Input: part model. Units: mm. Frame: model coordinates. Face numbers are marked on the shaded views. A direction names the side the tool comes from. Coordinates: 2 decimals unless noted, no trailing zeros. Loops run counter-clockwise (first coordinate to the right, second up) from the corner with the lowest first, then second, coordinate; pieces in that order, holes last. Notation, with made-up numbers: (14.25, 26) -> (42.25, 26) arc R30 cw to (42.25, 56) -> close; hole circle Ø1 at (-17, -35). An arc over 180 degrees is marked (long way). Put each result on its own line as item: value. Start each with the question number.
1) Cut plane A-A (x = -4.5). Return the cut outline in (y, z).
2) Set-up query: the marked faces 1, 2 and 3. Return all of +Z, -Z, +X, -X, +Y, -Y with unobstructed straight access to the full face (end or side cutting, diameter ignored); none if empty.
3) Material intervals for L1, parallel to Z at x = -5.5, y = 10.5; L2, parallel to Y at x = 13, z = 2; L3, parallel to Z at x = 7, y = 4, sorted ascending.
4) Cut plane C-C (z = 44). Return the cut outline in (x, y).
5) Cut plane D-D (z = 76). Return the cut outline in (x, y).
6) Contact query for flat-ended pins moving along their axis: P1, Ø12, axis at x = 10, z = 90.5, coming from the +Y side; P2, Ø6, axis at x = 5, y = -4, coming from the -Z side; P3, Ø16, axis at x = -4.5, y = 2, coming from the -Z side; P4, Ø2, axis at y = -3, z = 20.5, coming from the -X side. Output: stop coordinate, or through.
7) Cut plane B-B (y = -5). Return the cut outline in (x, z), plus the area to 3 significant figures.
from build123d import *

# Parameters (mm, degrees)
SKETCH1_R           = 16
BOSS_EXTRUDE1_DEPTH = 67.5
SKETCH2_R           = 9
BOSS_EXTRUDE2_DEPTH = 1
SKETCH3_R           = 3
BOSS_EXTRUDE3_DEPTH = 21
CUT_EXTRUDE1_DEPTH  = 17.698
SKETCH5_R           = 11
BOSS_EXTRUDE4_DEPTH = 39
CIRPATTERN1_COUNT   = 4


with BuildPart() as part:
    # Sketch1 → Boss-Extrude1 (new body)
    with BuildSketch(Plane.XY):
        Circle(SKETCH1_R)
    extrude(amount=BOSS_EXTRUDE1_DEPTH)

    # Sketch2 → Boss-Extrude2 (add)
    with BuildSketch(Plane(origin=(0, 0, 0), x_dir=(-1, 0, 0), z_dir=(0, 0, -1))):
        with Locations(Location((0, 0, 0), (0, 0, 180))):
            Circle(SKETCH2_R)
    extrude(amount=BOSS_EXTRUDE2_DEPTH)

    # Sketch3 → Boss-Extrude3 (add)
    with BuildSketch(Plane(origin=(0, 0, -1), x_dir=(-1, 0, 0), z_dir=(0, 0, -1))):
        with Locations(Location((0, 0, 0), (0, 0, 180))):
            Circle(SKETCH3_R)
    extrude(amount=BOSS_EXTRUDE3_DEPTH)

    # Sketch4 → Cut-Extrude1 (cut)
    with BuildSketch(Plane(origin=(0, 0, -22), x_dir=(-1, 0, 0), z_dir=(0, 0, -1))):
        Polygon((-3.161861974, 2.187315475), (3.465054218, 2.187315475), (3.465054218, 5.609056515), align=None)
    extrude(amount=-CUT_EXTRUDE1_DEPTH, mode=Mode.SUBTRACT)

    # Sketch5 → Boss-Extrude4 (add)
    with BuildSketch(Plane.XY.offset(67.5)):
        Circle(SKETCH5_R)
    extrude(amount=BOSS_EXTRUDE4_DEPTH)

    # Sketch8 → M3x0.5 Tapped Hole1 (revolve, cut)
    with BuildSketch(Plane(origin=(0, 13, 0), x_dir=(0, 1, 0), z_dir=(1, 0, 0))):
        Polygon((0, 0), (0, 8.371075774), (1.25, 7.62), (1.25, 0), align=None)
    m3x0_5_tapped_hole1 = revolve(axis=Axis((0, 13, -6.35), (0, 0, 1)), mode=Mode.SUBTRACT)

    # CirPattern1: M3x0.5 Tapped Hole1 ×4 about axis
    cirpattern1_axis = Axis((0, 0, 0), (0, 0, 1))
    for i in range(1, CIRPATTERN1_COUNT):
        add(m3x0_5_tapped_hole1.rotate(cirpattern1_axis, i * 360 / CIRPATTERN1_COUNT), mode=Mode.SUBTRACT)


solid = part.part
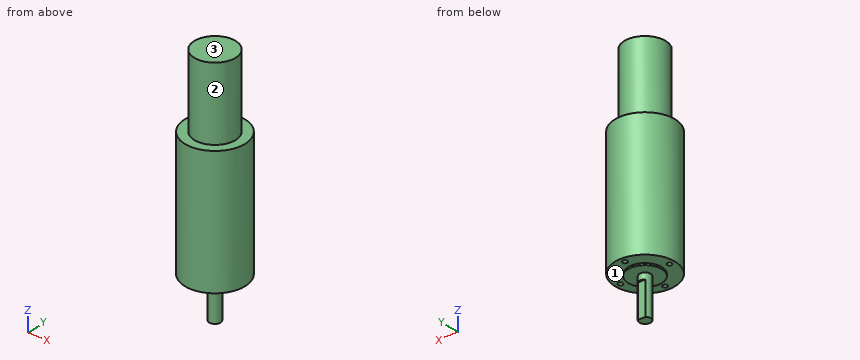
Results found:
1. outline: (-15.35, 0) -> (-7.79, 0) -> (-7.79, -1) -> (7.79, -1) -> (7.79, 0) -> (15.35, 0) -> (15.35, 67.5) -> (10.04, 67.5) -> (10.04, 106.5) -> (-10.04, 106.5) -> (-10.04, 67.5) -> (-15.35, 67.5) -> close
2. face 1: -Z
2. face 2: +Z
2. face 3: +Z, +X, -X, +Y, -Y
3. L1: z = 0 to 67.5
3. L2: y = -9.33 to -1.25, 1.25 to 9.33
3. L3: z = -1 to 106.5
4. outline: circle Ø32 at (0, 0)
5. outline: circle Ø22 at (0, 0)
6. P1: stops at y = 10.25
6. P2: stops at z = -1
6. P3: stops at z = -22
6. P4: stops at x = -15.87
7. outline: (-15.2, 0) -> (-7.48, 0) -> (-7.48, -1) -> (7.48, -1) -> (7.48, 0) -> (15.2, 0) -> (15.2, 67.5) -> (9.8, 67.5) -> (9.8, 106.5) -> (-9.8, 106.5) -> (-9.8, 67.5) -> (-15.2, 67.5) -> close
7. area: 2,830 mm2
